The listing builds one solid part. Answer for the finished solid, in the listing's coordinates (mm). A direction names the side the tool comes from. Give positions to 0.01 mm unless a question says otherwise; leave off trailing zeros. Write each loop counter-clockwise with the first axis right and the second up, starting at its lowest first coordinate (ties: lowest second). Pieces come first, ordered by that corner, then holes. Notation, with made-up numbers: (-8, 11) - (23, 11) arc R24 cw to (23, 41) - close; hole circle Ø9 at (-31, 31.25). An arc over 180 degrees is marked (long way). Return JSON: item names as keys, results as strings.
from build123d import *

# Parameters (mm, degrees)
SKETCH1_R           = 1.778
BOSS_EXTRUDE1_DEPTH = 2.54
FILLET1_R           = 2.54
BOSS_EXTRUDE2_START = -15.24
SKETCH3_R           = 42.173631202
SKETCH3_R_2         = 38.557688222
SKETCH3_R_3         = 1.778
BOSS_EXTRUDE2_DEPTH = 15.24
SKETCH4_R           = 42.173631202
BOSS_EXTRUDE3_DEPTH = 2.54


with BuildPart() as part:
    # Sketch1 → Boss-Extrude1 (new, symmetric)
    with BuildSketch(Plane.XY):
        with BuildLine():
            ThreePointArc((23.096897519, 13.335), (18.163878776, 19.528502447), (11.629866574, 24.000731311))
            add(Edge.make_bspline(
                [(12.942718979, 26.367649013), (12.489890773, 26.524403161), (10.214611, 26.823602727), (8.514999239, 25.805149786), (11.629866574, 24.000731311)],
                knots=[0.119187678, 0.119187678, 0.119187678, 0.119187678, 0.354139338, 1, 1, 1, 1], degree=3))
            ThreePointArc((12.942718979, 26.367649013), (14.594299506, 26.395047723), (14.579783558, 28.046791715))
            ThreePointArc((14.579783558, 28.046791715), (0, 32.207688222), (-14.579783558, 28.046791715))
            ThreePointArc((-14.579783558, 28.046791715), (-14.594299506, 26.395047723), (-12.942718979, 26.367649013))
            add(Edge.make_bspline(
                [(-12.942718979, 26.367649013), (-12.489890773, 26.524403161), (-10.214611, 26.823602727), (-8.514999239, 25.805149786), (-11.629866574, 24.000731311)],
                knots=[0.119187678, 0.119187678, 0.119187678, 0.119187678, 0.354139338, 1, 1, 1, 1], degree=3))
            ThreePointArc((-11.629866574, 24.000731311), (-18.163878776, 19.528502447), (-23.096897519, 13.335))
            ThreePointArc((-23.096897519, 13.335), (-23.564242622, 12.49061126), (-24.000731311, 11.629866574))
            add(Edge.make_bspline(
                [(-26.367649013, 12.942718979), (-26.524403161, 12.489890773), (-26.823602727, 10.214611), (-25.805149786, 8.514999239), (-24.000731311, 11.629866574)],
                knots=[0.119187678, 0.119187678, 0.119187678, 0.119187678, 0.354139338, 1, 1, 1, 1], degree=3))
            ThreePointArc((-26.367649013, 12.942718979), (-26.395047723, 14.594299506), (-28.046791715, 14.579783558))
            ThreePointArc((-28.046791715, 14.579783558), (-32.207688222, 0), (-28.046791715, -14.579783558))
            ThreePointArc((-28.046791715, -14.579783558), (-26.395047723, -14.594299506), (-26.367649013, -12.942718979))
            add(Edge.make_bspline(
                [(-26.367649013, -12.942718979), (-26.524403161, -12.489890773), (-26.823602727, -10.214611), (-25.805149786, -8.514999239), (-24.000731311, -11.629866574)],
                knots=[0.119187678, 0.119187678, 0.119187678, 0.119187678, 0.354139338, 1, 1, 1, 1], degree=3))
            ThreePointArc((-24.000731311, -11.629866574), (-18.858537854, -18.858537854), (-11.629866574, -24.000731311))
            add(Edge.make_bspline(
                [(-12.942718979, -26.367649013), (-12.489890773, -26.524403161), (-10.214611, -26.823602727), (-8.514999239, -25.805149786), (-11.629866574, -24.000731311)],
                knots=[0.119187678, 0.119187678, 0.119187678, 0.119187678, 0.354139338, 1, 1, 1, 1], degree=3))
            ThreePointArc((-12.942718979, -26.367649013), (-14.594299506, -26.395047723), (-14.579783558, -28.046791715))
            ThreePointArc((-14.579783558, -28.046791715), (0, -32.207688222), (14.579783558, -28.046791715))
            ThreePointArc((14.579783558, -28.046791715), (14.594299506, -26.395047723), (12.942718979, -26.367649013))
            add(Edge.make_bspline(
                [(12.942718979, -26.367649013), (12.489890773, -26.524403161), (10.214611, -26.823602727), (8.514999239, -25.805149786), (11.629866574, -24.000731311)],
                knots=[0.119187678, 0.119187678, 0.119187678, 0.119187678, 0.354139338, 1, 1, 1, 1], degree=3))
            ThreePointArc((11.629866574, -24.000731311), (18.858537854, -18.858537854), (24.000731311, -11.629866574))
            add(Edge.make_bspline(
                [(26.367649013, -12.942718979), (26.524403161, -12.489890773), (26.823602727, -10.214611), (25.805149786, -8.514999239), (24.000731311, -11.629866574)],
                knots=[0.119187678, 0.119187678, 0.119187678, 0.119187678, 0.354139338, 1, 1, 1, 1], degree=3))
            ThreePointArc((26.367649013, -12.942718979), (26.395047723, -14.594299506), (28.046791715, -14.579783558))
            ThreePointArc((28.046791715, -14.579783558), (32.207688222, 0), (28.046791715, 14.579783558))
            ThreePointArc((28.046791715, 14.579783558), (26.395047723, 14.594299506), (26.367649013, 12.942718979))
            add(Edge.make_bspline(
                [(26.367649013, 12.942718979), (26.524403161, 12.489890773), (26.823602727, 10.214611), (25.805149786, 8.514999239), (24.000731311, 11.629866574)],
                knots=[0.119187678, 0.119187678, 0.119187678, 0.119187678, 0.354139338, 1, 1, 1, 1], degree=3))
            ThreePointArc((24.000731311, 11.629866574), (23.564242622, 12.49061126), (23.096897519, 13.335))
        make_face()
        with Locations((0, 17.78)):
            Circle(SKETCH1_R, mode=Mode.SUBTRACT)
        with Locations((15.397931679, -8.89)):
            Circle(SKETCH1_R, mode=Mode.SUBTRACT)
        with Locations((-15.397931679, -8.89)):
            Circle(SKETCH1_R, mode=Mode.SUBTRACT)
        with BuildLine():
            Line((-4.28625, 20.274952091), (-4.28625, 22.454568821))
            ThreePointArc((-4.28625, 22.454568821), (-13.24349331, 18.633021359), (-19.797340731, 11.43))
            ThreePointArc((-19.797340731, 11.43), (-22.758416501, 2.152690962), (-21.58935203, -7.515283024))
            Line((-21.58935203, -7.515283024), (-17.877685951, -4.59493961))
            ThreePointArc((-17.877685951, -4.59493961), (-10.605148477, -7.614870918), (-15.415498572, -13.849477433))
            Line((-15.415498572, -13.849477433), (-17.30310203, -14.939285797))
            ThreePointArc((-17.30310203, -14.939285797), (-9.514923191, -20.78571232), (0, -22.86))
            ThreePointArc((0, -22.86), (9.514923191, -20.78571232), (17.30310203, -14.939285797))
            Line((17.30310203, -14.939285797), (12.918177407, -13.18506039))
            ThreePointArc((12.918177407, -13.18506039), (11.8972459, -5.376892533), (19.701748572, -6.425474659))
            Line((19.701748572, -6.425474659), (21.58935203, -7.515283024))
            ThreePointArc((21.58935203, -7.515283024), (22.758416501, 2.152690962), (19.797340731, 11.43))
            ThreePointArc((19.797340731, 11.43), (13.24349331, 18.633021359), (4.28625, 22.454568821))
            Line((4.28625, 22.454568821), (4.959508544, 17.78))
            ThreePointArc((4.959508544, 17.78), (-1.292097423, 12.991763451), (-4.28625, 20.274952091))
        make_face(mode=Mode.SUBTRACT)
    extrude(amount=BOSS_EXTRUDE1_DEPTH, both=True)

    # Fillet1
    # the kernel refuses this fillet: 2.54 mm, written as the material it adds along each edge
    with BuildSketch(Plane(origin=(21.58935203, -7.515283024, 0), x_dir=(-0.8660254037844372, 0.5000000000000026, 0), z_dir=(0, 0, -1)), Plane(origin=(-17.30310203, -14.939285797, 0), x_dir=(0.8660254037844382, 0.5000000000000008, 0), z_dir=(0, 0, -1)), Plane(origin=(-4.28625, 22.454568821, 0), x_dir=(0, -1, 0), z_dir=(0, 0, -1))) as fillet1_piece_1:
        with BuildLine():
            CenterArc((3.235105636, 2.310312353), FILLET1_R, 161.0565991, 84.38964425)
            Line((0.832672738, 3.134882647), (0.78462408, 3.151374053))
            ThreePointArc((0.78462408, 3.151374053), (0.311567983, 1.595269408), (-0.049899042, 0.009525))
            Line((-0.049899042, 0.009525), (0, -0.0508))
            ThreePointArc((0, -0.0508), (1.089808365, -0.0508), (2.158506952, -0.046206247))
            Line((2.158506952, -0.046206247), (2.17961673, 0))
        make_face()
    extrude(amount=2.54)
    with BuildSketch(Plane(origin=(17.30310203, -14.939285797, 0), x_dir=(-0.7195709341275718, -0.6944189447003685, 0), z_dir=(0, 0, -1)), Plane(origin=(4.28625, 22.454568821, 0), x_dir=(0.9611699140434871, -0.2759572364291899, 0), z_dir=(0, 0, -1)), Plane(origin=(-21.58935203, -7.515283024, 0), x_dir=(-0.24159897991591575, 0.9703761811295601, 0), z_dir=(0, 0, -1))) as fillet1_piece_2:
        with BuildLine():
            CenterArc((3.922629513, 2.529497521), FILLET1_R, 155.785220789, 119.426923656)
            Line((1.60611307, 3.571299597), (1.559782741, 3.592135639))
            Line((1.559782741, 3.592135639), (-0.046330329, 0.020836042))
            Line((-0.046330329, 0.020836042), (-0.004614858, -0.05058995))
            ThreePointArc((-0.004614858, -0.05058995), (2.076686213, -0.145322312), (4.157987284, -0.05058995))
            Line((4.157987284, -0.05058995), (4.153372426, 0))
        make_face()
    extrude(amount=2.54)
    with BuildSketch(Plane(origin=(-21.58935203, -7.515283024, 0), x_dir=(-0.24159897991591575, 0.9703761811295601, 0), z_dir=(0, 0, 1)), Plane(origin=(4.28625, 22.454568821, 0), x_dir=(0.9611699140434871, -0.2759572364291899, 0), z_dir=(0, 0, 1)), Plane(origin=(17.30310203, -14.939285797, 0), x_dir=(-0.7195709341275718, -0.6944189447003685, 0), z_dir=(0, 0, 1))) as fillet1_piece_3:
        with BuildLine():
            CenterArc((3.922629513, -2.529497521), FILLET1_R, 84.787855555, 119.426923656)
            Line((1.60611307, -3.571299597), (1.559782741, -3.592135639))
            Line((1.559782741, -3.592135639), (-0.046330329, -0.020836042))
            Line((-0.046330329, -0.020836042), (-0.004614858, 0.05058995))
            ThreePointArc((-0.004614858, 0.05058995), (2.076686213, 0.145322312), (4.157987284, 0.05058995))
            Line((4.157987284, 0.05058995), (4.153372426, 0))
        make_face()
    extrude(amount=2.54)
    with BuildSketch(Plane(origin=(-4.28625, 22.454568821, 0), x_dir=(0, -1, 0), z_dir=(0, 0, 1)), Plane(origin=(-17.30310203, -14.939285797, 0), x_dir=(0.8660254037844382, 0.5000000000000008, 0), z_dir=(0, 0, 1)), Plane(origin=(21.58935203, -7.515283024, 0), x_dir=(-0.8660254037844372, 0.5000000000000026, 0), z_dir=(0, 0, 1))) as fillet1_piece_4:
        with BuildLine():
            CenterArc((3.235105636, -2.310312353), FILLET1_R, 114.55375665, 84.38964425)
            Line((0.832672738, -3.134882647), (0.78462408, -3.151374053))
            ThreePointArc((0.78462408, -3.151374053), (0.311567983, -1.595269408), (-0.049899042, -0.009525))
            Line((-0.049899042, -0.009525), (0, 0.0508))
            ThreePointArc((0, 0.0508), (1.089808365, 0.0508), (2.158506952, 0.046206247))
            Line((2.158506952, 0.046206247), (2.17961673, 0))
        make_face()
    extrude(amount=2.54)

    # Sketch3 → Boss-Extrude2 (add)
    # profile 1 of 4: a face of its own
    with BuildSketch(Plane.XY.offset(2.54).offset(BOSS_EXTRUDE2_START)):
        Circle(SKETCH3_R)
        Circle(SKETCH3_R_2, mode=Mode.SUBTRACT)
    # profile 2 of 4: a face of its own
    with BuildSketch(Plane.XY.offset(2.54).offset(BOSS_EXTRUDE2_START)):
        with Locations((15.397931679, -8.89)):
            Circle(SKETCH3_R_3)
    # profile 3 of 4: a face of its own
    with BuildSketch(Plane.XY.offset(2.54).offset(BOSS_EXTRUDE2_START)):
        with Locations((-15.397931679, -8.89)):
            Circle(SKETCH3_R_3)
    # profile 4 of 4: a face of its own
    with BuildSketch(Plane.XY.offset(2.54).offset(BOSS_EXTRUDE2_START)):
        with Locations((0, 17.78)):
            Circle(SKETCH3_R_3)
    extrude(amount=BOSS_EXTRUDE2_DEPTH)


with BuildPart() as boss_extrude2_piece_1:
    # of the separate pieces the step leaves, piece 1, a body of its own (boss_extrude2_pieces)
    add(part.part.solids().sort_by_distance((42.173631202, 0, -12.7))[0])



with BuildPart() as boss_extrude2_piece_2:
    # of the separate pieces the step leaves, piece 2, a body of its own (boss_extrude2_pieces)
    add(part.part.solids().sort_by_distance((-18.511883244, -5.093926817, -2.54))[0])


with BuildPart() as boss_extrude2_piece_1_1:
    add(boss_extrude2_piece_1.part)

    add(boss_extrude2_piece_2.part)  # Boss-Extrude3 merges Boss-Extrude2 piece 2
    # Sketch4 → Boss-Extrude3 (add)
    with BuildSketch(Plane.XY.offset(2.54)):
        Circle(SKETCH4_R)
    extrude(amount=BOSS_EXTRUDE3_DEPTH)


solid = boss_extrude2_piece_1_1.part
Item 1: For faces 1 (the face through (17.79, -34.21, -5.19)), 2 (the face through (-15, -9, -12.7)), determine the directions among +Z, -Z, +X, -X, +Y, -Y from which every point of the face is accessible in a straight line to the end or side of a thin tool.
Answer below:
{"face 1": "-Z", "face 2": "-Z, +X, -X, +Y, -Y"}
Item 2: A cutting plane is placed at C-C on y = 0. Determine the outline of the cut face in (x, z).
Answer below:
{"outline": "(-42.17, -12.7) - (-38.56, -12.7) - (-38.56, 2.54) - (-32.21, 2.54) - (-32.21, -2.54) - (-22.86, -2.54) - (-22.86, 2.54) - (22.86, 2.54) - (22.86, -2.54) - (32.21, -2.54) - (32.21, 2.54) - (38.56, 2.54) - (38.56, -12.7) - (42.17, -12.7) - (42.17, 5.08) - (-42.17, 5.08) - close"}
Item 3: Flat-ended cylindrical pins translate along their axes: P1, Ø5, axis at x = -23.5, z = -4, coming from the +Y side; P2, Ø1.5, axis at x = -1.5, z = -9.5, coming from the -Y side; P3, Ø1, axis at x = 2.5, z = -10.5, coming from the -Y side. Find the tip coordinate at first contact, or state that the pin passes through.
Answer below:
{"P1": "stops at y = 36.57", "P2": "stops at y = -42.17", "P3": "stops at y = -42.13"}
Item 4: A cutting plane is placed at D-D on x = -30.5. Determine the outline of the cut face in (y, z).
Answer below:
{"outline": "(-29.13, -12.7) - (-23.59, -12.7) - (-23.59, 2.54) - (-9.56, 2.54) - (-9.56, -2.54) - (9.56, -2.54) - (9.56, 2.54) - (23.59, 2.54) - (23.59, -12.7) - (29.13, -12.7) - (29.13, 5.08) - (-29.13, 5.08) - close"}
Item 5: A cutting plane is placed at A-A on z = -5.25. Determine the outline of the cut face in (x, y).
Answer below:
{"outline": "circle Ø84.35 at (0, 0); circle Ø3.56 at (-15.4, -8.89); circle Ø3.56 at (0, 17.78); circle Ø3.56 at (15.4, -8.89); hole circle Ø77.12 at (0, 0)"}
Item 6: A cutting plane is placed at B-B on x = 0. Determine the outline of the cut face in (y, z).
Answer below:
{"outline": "(-42.17, -12.7) - (-38.56, -12.7) - (-38.56, 2.54) - (-32.21, 2.54) - (-32.21, -2.54) - (-22.86, -2.54) - (-22.86, 2.54) - (12.82, 2.54) - (12.82, -2.54) - (16, -2.54) - (16, -12.7) - (19.56, -12.7) - (19.56, -2.54) - (32.21, -2.54) - (32.21, 2.54) - (38.56, 2.54) - (38.56, -12.7) - (42.17, -12.7) - (42.17, 5.08) - (-42.17, 5.08) - close"}
Item 7: Consider L1, parallel to Y at x = 0, z = -9.5; L2, parallel to Y at x = -8.5, z = 2; L3, parallel to X at y = -23.5, z = -2.5. Determine where each line is inside the solid, lowest interval first.
Answer below:
{"L1": "y = -42.17 to -38.56, 16 to 19.56, 38.56 to 42.17", "L2": "y = -41.31 to -37.61, -30.87 to -21.22, 21.22 to 30.87, 37.61 to 41.31", "L3": "x = -35.02 to -30.57, -12.61 to 12.61, 30.57 to 35.02"}
Item 8: The mould has two halves that part along Y. Classify faces 3 (the face through (-18.947, -18.77, 0.036)), 4 (the face through (34, -19, -12.7)): +Y half, -Y half, draft (parallel to the pull), parting line (faces both ways), or undercut.
Answer below:
{"face 3": "undercut", "face 4": "draft"}
